Source: CAD feature listing. Evaluate the final solid. Frame: model axes, mm. Give positions to 0.01 mm unless a question says otherwise; leave off trailing zeros. Loops run counter-clockwise (first coordinate to the right, second up) from the corner with the lowest first, then second, coordinate; pieces in that order, holes last. Notation, with made-up numbers: (73.25, 15) -> (90.25, 15) arc R8 ccw to (90.25, 20) -> close; hole circle Ø10 at (59, 88.25). An arc over 180 degrees is marked (long way). Return JSON: item names as keys, results as strings. Group by question number.
(1) Cut plane A-A on z = 49. Return loops of the section in (x, y), then the cut area to 3 significant figures.
(2) Pin query (flat end, axial travel): pin 1 (12 mm diameter, centred on x = 22, z = 110.5, fed in from +Y). Return the tip coordinate at first contact, or that it passes through.
(3) Ray query, line 1 (X direction, y = -0.9, z = 84.5); line 2 (X direction, y = -1.15, z = 201.5); line 3 (Z direction, x = 37, y = -1.45). Return the intervals inside material, ascending. Write a range as from..to.
(4) Cut plane C-C on y = -1.15. Give the number of separate pieces and of enclosed holes in the cut face, then the cut area to 3 significant figures.
(5) Cut plane B-B on x = 25. Return loops of the section in (y, z).
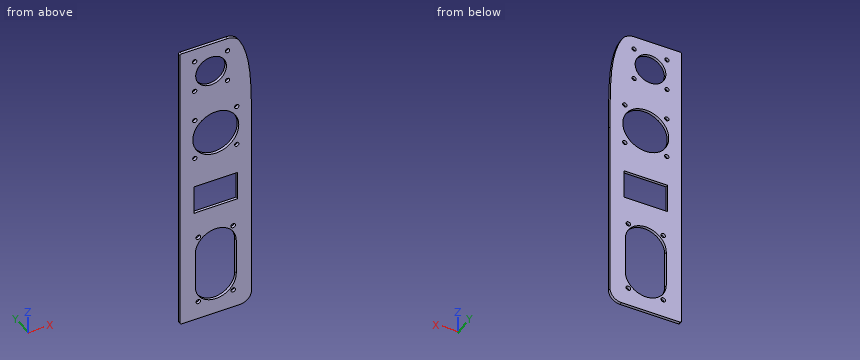
```python
from build123d import *

# Parameters (mm, degrees)
F0_R     = 1.6
F0_W     = 30.7
F0_H     = 20.5
F0_R_2   = 1.524
F0_R_3   = 16.1
F0_R_4   = 10.75
F1_DEPTH = 2


with BuildPart() as f1:
    # F0 (on Front) → F1 (new body)
    with BuildSketch(Plane.XZ):
        with BuildLine():
            ThreePointArc((0, 1), (0.292893, 0.292893), (1, 0))
            Line((1, 0), (42, 0))
            ThreePointArc((42, 0), (47.656854, 2.343146), (50, 8))
            Line((50, 8), (50, 133.995056))
            add(Edge.make_bspline(
                [(41.786822, 204.882652), (50, 190.202921), (50, 167.68368), (50, 133.995056)],
                knots=[8.50185, 8.50185, 8.50185, 8.50185, 76.896032, 76.896032, 76.896032, 76.896032], degree=3))
            ThreePointArc((41.786822, 204.882652), (38.118203, 208.626312), (33.059869, 210))
            Line((33.059869, 210), (1, 210))
            ThreePointArc((1, 210), (0.292893, 209.707107), (0, 209))
            Line((0, 209), (0, 1))
        make_face()
        with Locations((12.8, 13)):
            Circle(F0_R, mode=Mode.SUBTRACT)
        with BuildLine():
            ThreePointArc((39.35, 25.15), (25, 10.8), (10.65, 25.15))
            Line((10.65, 25.15), (10.65, 50.85))
            ThreePointArc((10.65, 50.85), (25, 65.2), (39.35, 50.85))
            Line((39.35, 50.85), (39.35, 25.15))
        make_face(mode=Mode.SUBTRACT)
        with Locations((12.8, 63)):
            Circle(F0_R, mode=Mode.SUBTRACT)
        with Locations((25, 93)):
            Rectangle(F0_W, F0_H, mode=Mode.SUBTRACT)
        with Locations((37.2, 13)):
            Circle(F0_R, mode=Mode.SUBTRACT)
        with Locations((37.2, 63)):
            Circle(F0_R, mode=Mode.SUBTRACT)
        with Locations((10.319, 125.319)):
            Circle(F0_R_2, mode=Mode.SUBTRACT)
        with Locations((10.319, 154.681)):
            Circle(F0_R_2, mode=Mode.SUBTRACT)
        with Locations((25, 140)):
            Circle(F0_R_3, mode=Mode.SUBTRACT)
        with Locations((10.194, 177.494)):
            Circle(F0_R_2, mode=Mode.SUBTRACT)
        with Locations((10.194, 200.506)):
            Circle(F0_R_2, mode=Mode.SUBTRACT)
        with Locations((21.7, 189)):
            Circle(F0_R_4, mode=Mode.SUBTRACT)
        with Locations((39.681, 125.319)):
            Circle(F0_R_2, mode=Mode.SUBTRACT)
        with Locations((39.681, 154.681)):
            Circle(F0_R_2, mode=Mode.SUBTRACT)
        with Locations((33.206, 177.494)):
            Circle(F0_R_2, mode=Mode.SUBTRACT)
        with Locations((33.206, 200.506)):
            Circle(F0_R_2, mode=Mode.SUBTRACT)
    extrude(amount=F1_DEPTH)


solid = f1.part
```
Answers:
{
 "1": {"outline": "(0, -2) -> (10.65, -2) -> (10.65, 0) -> (0, 0) -> close; (39.35, -2) -> (50, -2) -> (50, 0) -> (39.35, 0) -> close", "area": "42.6 mm²"},
 "2": {"pin 1": "y = 0"},
 "3": {"line 1": "0..9.65, 40.35..50", "line 2": "0..9.04, 11.35..32.05, 34.36..43.48", "line 3": "0..11.41, 14.59..17.28, 58.72..61.41, 64.59..82.75, 103.25..129.27, 150.73..209.19"},
 "4": {"separate pieces": "1", "enclosed holes": "16", "area": "7,040 mm²"},
 "5": {"outline": "(-2, 0) -> (0, 0) -> (0, 10.8) -> (-2, 10.8) -> close; (-2, 65.2) -> (0, 65.2) -> (0, 82.75) -> (-2, 82.75) -> close; (-2, 103.25) -> (0, 103.25) -> (0, 123.9) -> (-2, 123.9) -> close; (-2, 156.1) -> (0, 156.1) -> (0, 178.77) -> (-2, 178.77) -> close; (-2, 199.23) -> (0, 199.23) -> (0, 210) -> (-2, 210) -> close"}
}
